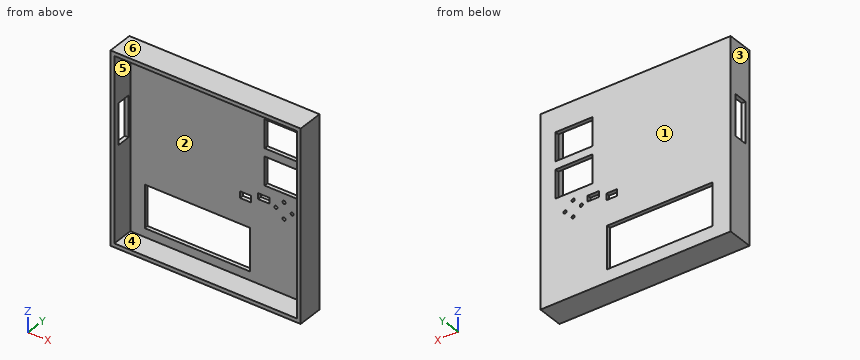
```python
from build123d import *

# Parameters (mm, degrees)
SKETCH1_W           = 94
SKETCH1_H           = 94
BOSS_EXTRUDE1_DEPTH = 12.7
SHELL3_T            = -1.905
SKETCH2_W           = 18.3
SKETCH2_H           = 14
SKETCH2_W_2         = 52
SKETCH2_H_2         = 21
CUT_EXTRUDE2_DEPTH  = 2.54
SKETCH2_11_R        = 0.762
CUT_EXTRUDE4_DEPTH  = 2.54
SKETCH2_12_W        = 5.216658821
SKETCH2_12_H        = 3.236828516
SKETCH2_12_W_2      = 5.589277308
SKETCH2_12_H_2      = 2.856741735
CUT_EXTRUDE5_DEPTH  = 2.54
SKETCH4_W           = 20.251250208
SKETCH4_H           = 6.910379218
CUT_EXTRUDE6_DEPTH  = 2.54


with BuildPart() as part:
    # Sketch1 → Boss-Extrude1 (new body)
    with BuildSketch(Plane(origin=(0, 0, 0), x_dir=(1, 0, 0), z_dir=(0, 1, 0))):
        with Locations((7.550289017, -23.555105973)):
            Rectangle(SKETCH1_W, SKETCH1_H)
    extrude(amount=BOSS_EXTRUDE1_DEPTH)

    # Shell3
    shell3_openings = [part.faces().sort_by_distance(p)[0] for p in [
        (7.550289017, 0, 23.555105973),
    ]]
    offset(amount=SHELL3_T, openings=shell3_openings, kind=Kind.INTERSECTION)

    # Sketch2 → Cut-Extrude2 (cut)
    with BuildSketch(Plane(origin=(0, 12.7, 0), x_dir=(1, 0, 0), z_dir=(0, 1, 0))):
        with Locations((38.011142824, -33.986529837)):
            Rectangle(SKETCH2_W, SKETCH2_H)
        with Locations((-4.438857176, 6.761825207)):
            Rectangle(SKETCH2_W_2, SKETCH2_H_2)
        with Locations((38.011142824, -51.906174793)):
            Rectangle(SKETCH2_W, SKETCH2_H)
    extrude(amount=-CUT_EXTRUDE2_DEPTH, mode=Mode.SUBTRACT)

    # Sketch2_11 → Cut-Extrude4 (cut)
    with BuildSketch(Plane(origin=(0, 12.7, 0), x_dir=(1, 0, 0), z_dir=(0, 1, 0))):
        with Locations(Location((38.411142824, -14.672051962, 0), (0, 0, 270))):
            Circle(SKETCH2_11_R)
        with Locations(Location((34.377019993, -18.706174793, 0), (0, 0, 270))):
            Circle(SKETCH2_11_R)
        with Locations(Location((38.411142824, -22.740297623, 0), (0, 0, 270))):
            Circle(SKETCH2_11_R)
        with Locations(Location((42.445265655, -18.706174793, 0), (0, 0, 270))):
            Circle(SKETCH2_11_R)
    extrude(amount=-CUT_EXTRUDE4_DEPTH, mode=Mode.SUBTRACT)

    # Sketch2_12 → Cut-Extrude5 (cut)
    with BuildSketch(Plane(origin=(0, 12.7, 0), x_dir=(1, 0, 0), z_dir=(0, 1, 0))):
        with Locations((19.369472235, -17.749589051)):
            Rectangle(SKETCH2_12_W, SKETCH2_12_H)
        with Locations((28.455781478, -20.607545661)):
            Rectangle(SKETCH2_12_W_2, SKETCH2_12_H_2)
    extrude(amount=-CUT_EXTRUDE5_DEPTH, mode=Mode.SUBTRACT)

    # Sketch4 → Cut-Extrude6 (cut)
    with BuildSketch(Plane.ZY.offset(39.449710983)):
        with Locations((34.355105973, 6.110056277)):
            Rectangle(SKETCH4_W, SKETCH4_H)
    extrude(amount=-CUT_EXTRUDE6_DEPTH, mode=Mode.SUBTRACT)


solid = part.part
```
Read the model definition and answer for the solid it produces. Units are mm, in the model's axes. Face numbers are marked on the shaded views. A direction names the side the tool comes from. Coordinates: 2 decimals unless noted, no trailing zeros. Write each loop counter-clockwise with the first axis right and the second up, starting at its lowest first coordinate (ties: lowest second). Pieces come first, ordered by that corner, then holes. Notation, with made-up numbers: (21, 78.5) -> (57, 78.5) arc R5 cw to (57, 87.5) -> close; hole circle Ø11 at (87, 7.25). An arc over 180 degrees is marked (long way). Write item = value, one per line.
(1) For a pull along X with two mould halves and no side action, classify the marked faces 3, 4, 5 and 6 as +X half, -X half, draft (parallel to the pull), parting line (faces both ways), or undercut.
From the geometry:
face_3 = -X half
face_4 = undercut
face_5 = undercut
face_6 = draft
(2) Section A-A on z = 34 is taken. Write down the section's boundary in (x, y) (3 decimals), plus the area to 3 significant figures.
From the geometry:
outline = (-39.45, 0) -> (-37.545, 0) -> (-37.545, 2.655) -> (-39.45, 2.655) -> close; (-39.45, 9.565) -> (-37.545, 9.565) -> (-37.545, 10.795) -> (28.861, 10.795) -> (28.861, 12.7) -> (-39.45, 12.7) -> close; (47.161, 10.795) -> (52.645, 10.795) -> (52.645, 0) -> (54.55, 0) -> (54.55, 12.7) -> (47.161, 12.7) -> close
area = 172 mm2
(3) Section C-C on x = 32.5 is taken. Write down the section's boundary in (y, z) (3 decimals), plus the area to 3 significant figures.
From the geometry:
outline = (0, -23.445) -> (12.7, -23.445) -> (12.7, 26.987) -> (10.795, 26.987) -> (10.795, -21.54) -> (0, -21.54) -> close; (0, 68.65) -> (10.795, 68.65) -> (10.795, 58.906) -> (12.7, 58.906) -> (12.7, 70.555) -> (0, 70.555) -> close; (10.795, 40.987) -> (12.7, 40.987) -> (12.7, 44.906) -> (10.795, 44.906) -> close
area = 167 mm2
(4) Section B-B on z = 54 is taken. Write down the section's boundary in (x, y) (3 decimals).
From the geometry:
outline = (-39.45, 0) -> (-37.545, 0) -> (-37.545, 10.795) -> (28.861, 10.795) -> (28.861, 12.7) -> (-39.45, 12.7) -> close; (47.161, 10.795) -> (52.645, 10.795) -> (52.645, 0) -> (54.55, 0) -> (54.55, 12.7) -> (47.161, 12.7) -> close
(5) Which of the six approach directions +Z, -Z, +X, -X, +Y, -Y give full straight-line access (tool end or side, diameter ignored) to the marked faces 1 and 2?
From the geometry:
face_1 = +Z, -Z, +X, -X, +Y
face_2 = -Y
(6) Section D-D on x = 5.5 is taken. Write down the section's boundary in (y, z) (3 decimals).
From the geometry:
outline = (0, -23.445) -> (12.7, -23.445) -> (12.7, -17.262) -> (10.795, -17.262) -> (10.795, -21.54) -> (0, -21.54) -> close; (0, 68.65) -> (10.795, 68.65) -> (10.795, 3.738) -> (12.7, 3.738) -> (12.7, 70.555) -> (0, 70.555) -> close
(7) Straight lines are drawn through the part: L1, parallel to X at y = 2.5, z = 45; L2, parallel to Z at x = 9, y = 7.5; L3, parallel to Z at x = 11, y = 11.5. For each, find the intervals that lie inside material, in ascending order. Write a range as from..to.
From the geometry:
L1 = -39.45..-37.54, 52.65..54.55
L2 = -23.44..-21.54, 68.65..70.56
L3 = -23.44..-17.26, 3.74..70.56
(8) Given pin 1 Ø4 at (x, z) = (20.5, -8.5) entering from -Y (3 decimals), flat-ended and moving along its own axis, determine where the tip first touches the part or whether it passes through.
From the geometry:
pin_1 = 10.795
